```python
from build123d import *

# Parameters (mm, degrees)
F1_DEPTH  = 25.4
F2_W      = 17.1734541655
F2_H      = 67.8351446986
F3_DEPTH  = 50.8
F4_R      = 8.3202188196
F5_DEPTH  = 34.036
F6_R      = 8.4229671273
F7_DEPTH  = 34.036
F8_R      = 7.7907761567
F9_DEPTH  = 38.2351304042
F10_W     = 15.4029955156
F10_H     = 18.5406394303
F11_DEPTH = 38.2351304042
F12_W     = 7.4162576348
F12_H     = 9.1277062893
F13_DEPTH = 38.2351304042
F14_R     = 3.6080391768
F15_DEPTH = 73.5484318443
F16_DEPTH = 73.5484318443
F17_R     = 3.2271301898
F18_DEPTH = 36.068


with BuildPart() as f1:
    # F0 (on Top) → F1 (new body)
    with BuildSketch(Plane.XY):
        with BuildLine():
            Line((-13.4350418075, 55.1854707301), (-0.6998389782, 55.1854707301))
            ThreePointArc((-0.6998389782, 55.1854707301), (-19.0618000925, 73.5474318443), (-37.4237612067, 55.1854707301))
            Line((-37.4237612067, 55.1854707301), (-24.6885583774, 55.1854707301))
            ThreePointArc((-24.6885583774, 55.1854707301), (-19.0618000925, 60.812229015), (-13.4350418075, 55.1854707301))
        make_face()
        with BuildLine():
            ThreePointArc((-37.4237612067, 55.1854707301), (-19.0618000925, 36.8235096158), (-0.6998389782, 55.1854707301))
            Line((-0.6998389782, 55.1854707301), (-13.4350418075, 55.1854707301))
            ThreePointArc((-13.4350418075, 55.1854707301), (-19.0618000925, 49.5587124451), (-24.6885583774, 55.1854707301))
            Line((-24.6885583774, 55.1854707301), (-37.4237612067, 55.1854707301))
        make_face()
        with BuildLine():
            ThreePointArc((-38.1236001849, -53.1297404909), (-19.0618000925, -36.0131404184), (0, -53.1297404909))
            Line((0, -53.1297404909), (0, 55.1854707301))
            Line((0, 55.1854707301), (-0.6998389782, 55.1854707301))
            ThreePointArc((-0.6998389782, 55.1854707301), (-19.0618000925, 36.8235096158), (-37.4237612067, 55.1854707301))
            Line((-37.4237612067, 55.1854707301), (-38.1236001849, 55.1854707301))
            Line((-38.1236001849, 55.1854707301), (-38.1236001849, -53.1297404909))
        make_face()
        with BuildLine():
            Line((-12.4822018454, -55.1854707301), (0, -55.1854707301))
            Line((0, -55.1854707301), (0, -53.1297404909))
            ThreePointArc((0, -53.1297404909), (-19.0618000925, -36.0131404184), (-38.1236001849, -53.1297404909))
            Line((-38.1236001849, -53.1297404909), (-38.1236001849, -55.1854707301))
            Line((-38.1236001849, -55.1854707301), (-25.6413983395, -55.1854707301))
            ThreePointArc((-25.6413983395, -55.1854707301), (-19.0618000925, -48.605872483), (-12.4822018454, -55.1854707301))
        make_face()
        with BuildLine():
            Line((0, -53.1297404909), (0, -55.1854707301))
            Line((0, -55.1854707301), (-12.4822018454, -55.1854707301))
            ThreePointArc((-12.4822018454, -55.1854707301), (-19.0618000925, -61.7650689771), (-25.6413983395, -55.1854707301))
            Line((-25.6413983395, -55.1854707301), (-38.1236001849, -55.1854707301))
            Line((-38.1236001849, -55.1854707301), (-38.1236001849, -53.1297404909))
            ThreePointArc((-38.1236001849, -53.1297404909), (-20.0911498563, -74.3301485452), (0.1105302192, -55.1854707301))
            ThreePointArc((0.1105302192, -55.1854707301), (0.0828777227, -54.1561209662), (0, -53.1297404909))
        make_face()
    extrude(amount=F1_DEPTH)

    # F2 (on Top) → F3 (join)
    with BuildSketch(Plane.XY):
        with Locations((-19.3063616753, 0)):
            Rectangle(F2_W, F2_H)
    extrude(amount=F3_DEPTH)

    # F4 (on Front) → F5 (join)
    with BuildSketch(Plane.XZ):
        with Locations((-19.4193646312, 50.8048012853)):
            Circle(F4_R)
    extrude(amount=F5_DEPTH)

    # F6 (on Front) → F7 (join)
    with BuildSketch(Plane.XZ):
        with Locations((-19.5526480675, 50.8048012853)):
            Circle(F6_R)
    extrude(amount=-F7_DEPTH)

    # F8 (on Right) → F9 (cut, through all)
    with BuildSketch(Plane.YZ):
        with Locations((0, 40.3615534306)):
            Circle(F8_R)
    extrude(amount=-F9_DEPTH, mode=Mode.SUBTRACT)

    # F10 (on Right) → F11 (cut, through all)
    with BuildSketch(Plane.YZ):
        with Locations((2.328e-07, 49.9171148986)):
            Rectangle(F10_W, F10_H)
    extrude(amount=-F11_DEPTH, mode=Mode.SUBTRACT)

    # F12 (on Right) → F13 (cut, through all)
    with BuildSketch(Plane.YZ):
        with Locations((3.7081288174, 60.043156147)):
            Rectangle(F12_W, F12_H)
    extrude(amount=-F13_DEPTH, mode=Mode.SUBTRACT)

    # F14 (on Front) → F15 (cut, through all)
    with BuildSketch(Plane.XZ):
        with Locations((-19.3963646889, 51.2006953359)):
            Circle(F14_R)
    extrude(amount=-F15_DEPTH, mode=Mode.SUBTRACT)

    # F14 (on Front) → F16 (cut, through all)
    with BuildSketch(Plane.XZ):
        with Locations((-19.3963646889, 51.2006953359)):
            Circle(F14_R)
    extrude(amount=-F16_DEPTH, mode=Mode.SUBTRACT)

    # F17 (on Front) → F18 (cut)
    with BuildSketch(Plane.XZ):
        with Locations((-19.3963646889, 51.2006953359)):
            Circle(F17_R)
    extrude(amount=F18_DEPTH, mode=Mode.SUBTRACT)


solid = f1.part
```
Verification items for the finished model (mm, model axes). A direction names the side the tool comes from. Round coordinates to 2 decimals unless told otherwise and drop trailing zeros. Write each loop counter-clockwise with the first axis right and the second up, starting at its lowest first coordinate (ties: lowest second). Pieces come first, ordered by that corner, then holes. Notation, with made-up numbers: (-36, -40) -> (-29, -40) arc R16 ccw to (-29, -13) -> close; hole circle Ø8 at (-37, 89.5). An arc over 180 degrees is marked (long way). Write each question's results on one line, items separated by ' | '. Start each with the question number.
1. Cross-section at B-B (y = -51). Enter the section's corners in (x, z), then the cut area to 3 significant figures.
2. Cross-section at C-C (z = 20.5). Enter the section's corners in (x, y), then the cut area to 3 significant figures.
3. Material ranges on probe 1 along Z at (x, y) = (-19.5, 18); probe 2 along Z at (x, y) = (-27.5, 52); probe 3 along X at (y, z) = (5.5, 7), recorded low to high. Write a range as from..to.
4. Set-up check for faces 4 (the flat face through (-38.124, 2, 13)), 5 (the cylindrical face through (-22.26, 20.684, 49.005)): record each of +Z, -Z, +X, -X, +Y, -Y from which the full face is reachable in a straight line by a thin tool's end or side.
5. Cross-section at D-D (y = -19). Enter the section's corners in (x, z).
6. Draft check along Z on faces 1 (the flat face through (-19, 33.918, 35)), 2 (the flat face through (-19, 1, 0)), 3 (the cylindrical face through (-24.683, 54.938, 12.522)). Enter one of: +Z half, -Z half, draft (parallel to the pull), parting line (faces both ways), or undercut.
7. Cross-section at A-A (z = 34.5). Enter the section's corners in (x, y), then the cut area to 3 significant figures.
8. Depth check by flat-ended pin: P1, Ø4, axis at y = 28, z = 13.5, coming from the -X side; P2, Ø13.5, axis at x = -16.5, z = 47, coming from the -Y side; P3, Ø7.5, axis at y = 16, z = 10, coming from the +X side; P4, Ø2, axis at x = -8.5, z = 27.5, coming from the +Y side. Enter the tip coordinate at first touch or a pass-through.
Solutions:
1) outline: (-38.12, 0) -> (-24.14, 0) -> (-24.14, 25.4) -> (-38.12, 25.4) -> close; (-13.99, 0) -> (0, 0) -> (0, 25.4) -> (-13.99, 25.4) -> close | area: 710 mm2
2) outline: (-38.12, -53.13) arc R19.17 ccw (long way) to (0, -53.13) -> (0, 55.19) -> (-0.7, 55.19) arc R18.36 ccw to (-37.42, 55.19) -> (-38.12, 55.19) -> close; hole circle Ø13.16 at (-19.06, -55.19); hole circle Ø11.25 at (-19.06, 55.19) | area: 5,080 mm2
3) probe 1: z = 0..47.59, 54.81..59.23 | probe 2: z = 0..25.4 | probe 3: x = -38.12..0
4) face 4: +Z, -Z, -X, +Y | face 5: +Y
5) outline: (-38.12, 0) -> (0, 0) -> (0, 25.4) -> (-10.72, 25.4) -> (-10.72, 50.8) -> (-11.1, 50.8) arc R8.32 ccw to (-27.74, 50.8) -> (-27.89, 50.8) -> (-27.89, 25.4) -> (-38.12, 25.4) -> close; hole circle Ø6.45 at (-19.4, 51.2)
6) face 1: undercut | face 2: -Z half | face 3: draft
7) outline: (-27.89, -33.92) -> (-10.72, -33.92) -> (-10.72, -5.13) -> (-27.89, -5.13) -> close; (-27.89, 5.13) -> (-10.72, 5.13) -> (-10.72, 33.92) -> (-27.89, 33.92) -> close | area: 989 mm2
8) P1: stops at x = -38.12 | P2: stops at y = -34.04 | P3: stops at x = 0 | P4: passes through
